```python
from build123d import *

# Parameters (mm, degrees)
SKETCH_1_W          = 67
SKETCH_1_H          = 30
EXTRUDE_1_DEPTH     = 5
SKETCH_3_R          = 11.5
CUT_EXTRUDE_1_DEPTH = 6
CUT_EXTRUDE_2_DEPTH = 5
EXTRUDE_2_DEPTH     = 5
FILLET_1_R          = 2.5
FILLET_3_R          = 0.5
FILLET_4_R          = 7
SKETCH_6_R          = 2
CUT_EXTRUDE_3_DEPTH = 6
EXTRUDE_3_DEPTH     = 5
CUT_EXTRUDE_4_DEPTH = 6
EXTRUDE_4_DEPTH     = 5
SKETCH_10_R         = 2.1
CUT_EXTRUDE_5_DEPTH = 6
FILLET_5_R          = 5
SKETCH_11_R         = 1.6
CUT_EXTRUDE_6_DEPTH = 6
CUT_EXTRUDE_7_DEPTH = 10
FILLET_6_R          = 2


with BuildPart() as part:
    # 草图1 → 凸台-拉伸1 (new body)
    with BuildSketch(Plane.XY):
        Rectangle(SKETCH_1_W, SKETCH_1_H)
    extrude(amount=EXTRUDE_1_DEPTH)

    # 草图3 → 切除-拉伸1 (cut, through all)
    with BuildSketch(Plane.XY.offset(5)):
        with Locations((0.155997342, -18.5)):
            Circle(SKETCH_3_R)
    extrude(amount=-CUT_EXTRUDE_1_DEPTH, mode=Mode.SUBTRACT)

    # 草图4 → 切除-拉伸2 (cut)
    with BuildSketch(Plane.XY.offset(5)):
        with BuildLine():
            Line((14.951296016, -3.246749948), (0.155997342, -34.975370344))
            Line((0.155997342, -34.975370344), (0.155997342, -27))
            Line((0.155997342, -27), (-20.283732192, -12.687947301))
            ThreePointArc((-20.283732192, -12.687947301), (-5.343907366, 2.025923809), (14.951296016, -3.246749948))
        make_face()
    extrude(amount=-CUT_EXTRUDE_2_DEPTH, mode=Mode.SUBTRACT)

    # 草图5 → 凸台-拉伸2 (add)
    with BuildSketch(Plane.XY.offset(5)):
        Polygon((-16.981778738, -15), (-2.700298671, -25), (-33.5, -25), (-33.5, -15), align=None)
        Polygon((33.5, -15), (33.5, -25), (4.807588927, -25), (10.334473164, -13.147558505), align=None)
    extrude(amount=-EXTRUDE_2_DEPTH)

    # 圆角1
    fillet_1_edges = [part.edges().sort_by_distance(p)[0] for p in [
        (-2.700298671, -25, 2.5),
    ]]
    fillet(fillet_1_edges, radius=FILLET_1_R)

    # 圆角3
    fillet_3_edges = [part.edges().sort_by_distance(p)[0] for p in [
        (14.951296016, -3.246749948, 2.5),
        (-20.283732192, -12.687947301, 2.5),
    ]]
    fillet(fillet_3_edges, radius=FILLET_3_R)

    # 圆角4
    fillet_4_edges = [part.edges().sort_by_distance(p)[0] for p in [
        (4.807588927, -25, 2.5),
    ]]
    fillet(fillet_4_edges, radius=FILLET_4_R)

    # 草图6 → 切除-拉伸3 (cut, through all)
    with BuildSketch(Plane.XY.offset(5)):
        with Locations((17.505658254, -13.841257188)):
            Circle(SKETCH_6_R)
        with Locations((-17.782400736, -20.381512339)):
            Circle(SKETCH_6_R)
    extrude(amount=-CUT_EXTRUDE_3_DEPTH, mode=Mode.SUBTRACT)

    # 草图7 → 凸台-拉伸3 (add)
    with BuildSketch(Plane.XY.offset(5)):
        Polygon((60.5, 75), (14.5, 75), (-16.303792618, 15), (33.5, 15), align=None)
    extrude(amount=-EXTRUDE_3_DEPTH)

    # 草图8 → 切除-拉伸4 (cut, through all)
    with BuildSketch(Plane.XY.offset(5)):
        Polygon((-16.303792618, 15), (-33.5, -18.49498082), (-33.5, 15), align=None)
    extrude(amount=-CUT_EXTRUDE_4_DEPTH, mode=Mode.SUBTRACT)

    # 草图9 → 凸台-拉伸4 (add)
    with BuildSketch(Plane.XY.offset(5)):
        Polygon((60.5, 75), (33.5, -25), (33.5, 15), align=None)
    extrude(amount=-EXTRUDE_4_DEPTH)

    # 草图10 → 切除-拉伸5 (cut, through all)
    with BuildSketch(Plane.XY.offset(5)):
        with Locations((-12, 10)):
            Circle(SKETCH_10_R)
        with Locations((23, 10)):
            Circle(SKETCH_10_R)
    extrude(amount=-CUT_EXTRUDE_5_DEPTH, mode=Mode.SUBTRACT)

    # 圆角5
    fillet_5_edges = [part.edges().sort_by_distance(p)[0] for p in [
        (60.5, 75, 2.5),
        (14.5, 75, 2.5),
    ]]
    fillet(fillet_5_edges, radius=FILLET_5_R)

    # 草图11 → 切除-拉伸6 (cut, through all)
    with BuildSketch(Plane.XY.offset(5)):
        with Locations((42.500000039, 67)):
            Circle(SKETCH_11_R)
        with Locations((22.500000039, 67)):
            Circle(SKETCH_11_R)
    extrude(amount=-CUT_EXTRUDE_6_DEPTH, mode=Mode.SUBTRACT)

    # 草图12 → 切除-拉伸7 (cut)
    with BuildSketch(Plane.XY.offset(5)):
        Polygon((33.412019277, 64), (31.452414539, 20), (29.670955687, -20), (52.350955687, 64), align=None)
        Polygon((28.047412755, 55.924590701), (-1.630833947, 20), (26.447458252, 20), align=None)
        Polygon((14.473082867, 64), (-8.116365053, 20), (28.233189094, 64), align=None)
    extrude(amount=-CUT_EXTRUDE_7_DEPTH, mode=Mode.SUBTRACT)

    # 圆角6
    fillet_6_edges = [part.edges().sort_by_distance(p)[0] for p in [
        (29.670955687, -20, 2.5),
        (33.412019277, 64, 2.5),
        (52.350955687, 64, 2.5),
        (14.473082867, 64, 2.5),
        (28.233189094, 64, 2.5),
        (-8.116365053, 20, 2.5),
        (28.047412755, 55.924590701, 2.5),
        (26.447458252, 20, 2.5),
        (-1.630833947, 20, 2.5),
    ]]
    fillet(fillet_6_edges, radius=FILLET_6_R)


solid = part.part
```
Part model, mm, in its own coordinate system. A direction names the side the tool comes from. Round coordinates to 2 decimals unless told otherwise and drop trailing zeros. Order: outer loops, then holes, each group sorted by start corner. A loop starts at its lowest first (then second) coordinate and runs counter-clockwise, first axis right, second up. Notation, with made-up numbers: M 69.5,-25 L 119.5,-25 A29 ccw 119.5,3 Z; hole C 70.25,33 d9. An arc over 180 degrees is marked long. Answer in a Markdown table with one row per item. Add a question column.
Q1. Mould opens along Y. For faces 1 (the face through (36, 75, 3)), 2 (the face through (46.326, 22.504, 2.535)), 3 (the face through (25.782, 62.881, 2.465)) say: +Y half, -Y half, draft (parallel to the pull), parting line (faces both ways), or undercut.
Q2. 3-axis set-ups, long thin cutter, end or side, ignore diameter. For faces 4 (the face through (-33.5, -22, 3)), 5 (the face through (43, 64, 3)): which of +Z, -Z, +X, -X, +Y, -Y reach the whole face in a straight line?
Q3. Wall check: L1, parallel to Y at x = 17, z = 2.3; L2, parallel to X at y = 67, z = 1.2; L3, parallel to Y at x = 22.5, z = 2.5. Give the ranges that are in metal, low to high. Write a range as from..to.
Q4. Pin check, flat tips, straight feed: pin 1 (3 mm diameter, centred on x = -1, z = 1, fed in from -Y); pin 2 (2 mm diameter, centred on y = 14, z = 4.5, fed in from +X). Stop position of each tip, or through.
Q5. Cut at A-A on y = 10. Give the cut face in (x, z).
Q6. Cut at D-D on x = 22.5. Give the cut face in (y, z).
Q7. Cut at B-B on x = 5. Give the cut face in (y, z), and give its area (3 significant figures).
Q8. Cut at C-C on y = 67. Give the cut face in (x, z), and give its area (3 significant figures).
Established:
| question | item | result |
|---|---|---|
| 1 | face 1 | +Y half |
| 1 | face 2 | -Y half |
| 1 | face 3 | undercut |
| 2 | face 4 | +Z, -Z, -X, +Y, -Y |
| 2 | face 5 | +Z, -Z |
| 3 | L1 | y = -25..-15.78, -11.91..20, 42.55..50.4, 64..74.97 |
| 3 | L2 | x = 10.39..20.9, 24.1..40.9, 44.1..58.34 |
| 3 | L3 | y = -25..7.96, 12.04..20, 49.21..57.06, 64..65.4, 68.6..75 |
| 4 | pin 1 | stops at y = 2.58 |
| 4 | pin 2 | stops at x = 44.3 |
| 5 | outline | M -18.87,0 L -14.1,0 L -14.1,5 L -18.87,5 Z; M -9.9,0 L 20.9,0 L 20.9,5 L -9.9,5 Z; M 25.1,0 L 31.01,0 L 31.01,5 L 25.1,5 Z; M 37.77,0 L 42.95,0 L 42.95,5 L 37.77,5 Z |
| 6 | outline | M -25,0 L 7.96,0 L 7.96,5 L -25,5 Z; M 12.04,0 L 20,0 L 20,5 L 12.04,5 Z; M 49.21,0 L 57.06,0 L 57.06,5 L 49.21,5 Z; M 64,0 L 65.4,0 L 65.4,5 L 64,5 Z; M 68.6,0 L 75,0 L 75,5 L 68.6,5 Z |
| 7 | outline | M 2.19,0 L 20,0 L 20,5 L 2.19,5 Z; M 28.03,0 L 35.88,0 L 35.88,5 L 28.03,5 Z; M 45.55,0 L 56.5,0 L 56.5,5 L 45.55,5 Z |
| 7 | area | 183 mm2 |
| 8 | outline | M 10.39,0 L 20.9,0 L 20.9,5 L 10.39,5 Z; M 24.1,0 L 40.9,0 L 40.9,5 L 24.1,5 Z; M 44.1,0 L 58.34,0 L 58.34,5 L 44.1,5 Z |
| 8 | area | 208 mm2 |
